Design review of the part built by this model. Coordinates are the model's own, in mm. A direction names the side the tool comes from. Coordinates: 2 decimals unless noted, no trailing zeros. Write each loop counter-clockwise with the first axis right and the second up, starting at its lowest first coordinate (ties: lowest second). Pieces come first, ordered by that corner, then holes. Notation, with made-up numbers: (88, -2) - (114, -2) arc R20 ccw to (114, 28) - close; hole circle Ø9 at (63.25, 32). An arc over 180 degrees is marked (long way). Answer as a JSON object with one key per item and string values.
```python
from build123d import *

# Parameters (mm, degrees)
EXTRUDE_1_DEPTH = 1000


with BuildPart() as part:
    # Model → Бобышка-Вытянуть1 (new body)
    with BuildSketch(Plane.XY):
        with BuildLine():
            Line((-45, 0.5), (-45, 26.894643722))
            ThreePointArc((-45, 26.894643722), (-44.817095334, 27.281232068), (-44.402197802, 27.384985164))
            Line((-44.402197802, 27.384985164), (-42.406593407, 26.996231342))
            ThreePointArc((-42.406593407, 26.996231342), (-42.114835557, 26.823857), (-42, 26.505033614))
            Line((-42, 26.505033614), (-42, 6.5))
            ThreePointArc((-42, 6.5), (-41.853553391, 6.146446609), (-41.5, 6))
            Line((-41.5, 6), (-38, 6))
            ThreePointArc((-38, 6), (-37.646446609, 6.146446609), (-37.5, 6.5))
            Line((-37.5, 6.5), (-37.5, 25.528955097))
            ThreePointArc((-37.5, 25.528955097), (-37.323527943, 25.910176385), (-36.918681319, 26.022298052))
            Line((-36.918681319, 26.022298052), (-34.923076923, 25.70247728))
            ThreePointArc((-34.923076923, 25.70247728), (-34.620222737, 25.533651691), (-34.5, 25.208429873))
            Line((-34.5, 25.208429873), (-34.5, 6.5))
            ThreePointArc((-34.5, 6.5), (-34.353553391, 6.146446609), (-34, 6))
            Line((-34, 6), (-30.5, 6))
            ThreePointArc((-30.5, 6), (-30.146446609, 6.146446609), (-30, 6.5))
            Line((-30, 6.5), (-30, 24.420745635))
            ThreePointArc((-30, 24.420745635), (-29.829835124, 24.796523217), (-29.435164835, 24.916524216))
            Line((-29.435164835, 24.916524216), (-27.43956044, 24.664537804))
            ThreePointArc((-27.43956044, 24.664537804), (-27.125687443, 24.499700959), (-27, 24.168204187))
            Line((-27, 24.168204187), (-27, 6.5))
            ThreePointArc((-27, 6.5), (-26.853553391, 6.146446609), (-26.5, 6))
            Line((-26.5, 6), (-23, 6))
            ThreePointArc((-23, 6), (-22.646446609, 6.146446609), (-22.5, 6.5))
            Line((-22.5, 6.5), (-22.5, 23.56623485))
            ThreePointArc((-22.5, 23.56623485), (-22.336023939, 23.936488698), (-21.951648352, 24.063891477))
            Line((-21.951648352, 24.063891477), (-19.956043956, 23.878890172))
            ThreePointArc((-19.956043956, 23.878890172), (-19.631233121, 23.718481187), (-19.5, 23.380826054))
            Line((-19.5, 23.380826054), (-19.5, 6.5))
            ThreePointArc((-19.5, 6.5), (-19.353553391, 6.146446609), (-19, 6))
            Line((-19, 6), (-15.5, 6))
            ThreePointArc((-15.5, 6), (-15.146446609, 6.146446609), (-15, 6.5))
            Line((-15, 6.5), (-15, 22.962558154))
            ThreePointArc((-15, 22.962558154), (-14.842100814, 23.327204603), (-14.468131868, 23.461541543))
            Line((-14.468131868, 23.461541543), (-12.472527473, 23.342910858))
            ThreePointArc((-12.472527473, 23.342910858), (-12.13686348, 23.187369337), (-12, 22.843666168))
            Line((-12, 22.843666168), (-12, 6.5))
            ThreePointArc((-12, 6.5), (-11.853553391, 6.146446609), (-11.5, 6))
            Line((-11.5, 6), (11.5, 6))
            ThreePointArc((11.5, 6), (11.853553391, 6.146446609), (12, 6.5))
            Line((12, 6.5), (12, 22.843666168))
            ThreePointArc((12, 22.843666168), (12.13686348, 23.187369337), (12.472527473, 23.342910858))
            Line((12.472527473, 23.342910858), (14.468131868, 23.461541543))
            ThreePointArc((14.468131868, 23.461541543), (14.842100814, 23.327204603), (15, 22.962558154))
            Line((15, 22.962558154), (15, 6.5))
            ThreePointArc((15, 6.5), (15.146446609, 6.146446609), (15.5, 6))
            Line((15.5, 6), (19, 6))
            ThreePointArc((19, 6), (19.353553391, 6.146446609), (19.5, 6.5))
            Line((19.5, 6.5), (19.5, 23.380826054))
            ThreePointArc((19.5, 23.380826054), (19.631233121, 23.718481187), (19.956043956, 23.878890172))
            Line((19.956043956, 23.878890172), (21.951648352, 24.063891477))
            ThreePointArc((21.951648352, 24.063891477), (22.336023939, 23.936488698), (22.5, 23.56623485))
            Line((22.5, 23.56623485), (22.5, 6.5))
            ThreePointArc((22.5, 6.5), (22.646446609, 6.146446609), (23, 6))
            Line((23, 6), (26.5, 6))
            ThreePointArc((26.5, 6), (26.853553391, 6.146446609), (27, 6.5))
            Line((27, 6.5), (27, 24.168204187))
            ThreePointArc((27, 24.168204187), (27.125687443, 24.499700959), (27.43956044, 24.664537804))
            Line((27.43956044, 24.664537804), (29.435164835, 24.916524216))
            ThreePointArc((29.435164835, 24.916524216), (29.829835124, 24.796523217), (30, 24.420745635))
            Line((30, 24.420745635), (30, 6.5))
            ThreePointArc((30, 6.5), (30.146446609, 6.146446609), (30.5, 6))
            Line((30.5, 6), (34, 6))
            ThreePointArc((34, 6), (34.353553391, 6.146446609), (34.5, 6.5))
            Line((34.5, 6.5), (34.5, 25.208429873))
            ThreePointArc((34.5, 25.208429873), (34.620222737, 25.533651691), (34.923076923, 25.70247728))
            Line((34.923076923, 25.70247728), (36.918681319, 26.022298052))
            ThreePointArc((36.918681319, 26.022298052), (37.323527943, 25.910176385), (37.5, 25.528955097))
            Line((37.5, 25.528955097), (37.5, 6.5))
            ThreePointArc((37.5, 6.5), (37.646446609, 6.146446609), (38, 6))
            Line((38, 6), (41.5, 6))
            ThreePointArc((41.5, 6), (41.853553391, 6.146446609), (42, 6.5))
            Line((42, 6.5), (42, 26.505033614))
            ThreePointArc((42, 26.505033614), (42.114835557, 26.823857), (42.406593407, 26.996231342))
            Line((42.406593407, 26.996231342), (44.402197802, 27.384985164))
            ThreePointArc((44.402197802, 27.384985164), (44.817095334, 27.281232068), (45, 26.894643722))
            Line((45, 26.894643722), (45, 0.5))
            ThreePointArc((45, 0.5), (44.853553391, 0.146446609), (44.5, 0))
            Line((44.5, 0), (-44.5, 0))
            ThreePointArc((-44.5, 0), (-44.853553391, 0.146446609), (-45, 0.5))
        make_face()
    extrude(amount=EXTRUDE_1_DEPTH)


solid = part.part
```
(1) The part is to be moulded in two halves that separate along X. For faces 1 (the face through (45, 14, 493)), 2 (the face through (37.5, 16, 493)), 3 (the face through (1, 5, 0)), say which applies: pulls with the +X half, pulls with the -X half, needs draft (parallel to the pull), parting line crosses it, or undercut.
Solved:
{"face 1": "pulls with the +X half", "face 2": "undercut", "face 3": "needs draft"}
(2) Take a section at A-A, the plane y = 16.25. Give the number of separate pieces and of enclosed holes in the cut face, and give its area (3 significant figures).
Solved:
{"separate pieces": "10", "enclosed holes": "0", "area": "30,000 mm^2"}
(3) Tool access review of faces 4 (the face through (1, 5, 1000)), 5 (the face through (30, 16, 493)): name each direction out of +Z, -Z, +X, -X, +Y, -Y from which nothing blocks a thin tool from reaching the whole face with its end or side.
Solved:
{"face 4": "+Z, +X, -X, +Y, -Y", "face 5": "+Z, -Z, +Y"}
(4) To check wall thickness, follow line 1 (Y direction, x = 39, z = 58.5); line 2 (Y direction, x = -12.5, z = 640). State the ranges of each line that lie inside material, in increasing order. Write a range as from..to.
Solved:
{"line 1": "y = 0..6", "line 2": "y = 0..23.34"}
(5) Take a section at B-B, the plane x = 0.5. Write out the cut boundary in (y, z).
Solved:
{"outline": "(0, 0) - (6, 0) - (6, 1000) - (0, 1000) - close"}
(6) For pin 1 (1.8 mm diameter, centred on x = 40, z = 722, fed in from +Y); pin 2 (4 mm diameter, centred on x = -24, z = 322, fed in from +Y), all flat-tipped, find the tip position at first contact; note any pin that passes through.
Solved:
{"pin 1": "stops at y = 6", "pin 2": "stops at y = 24.07"}
